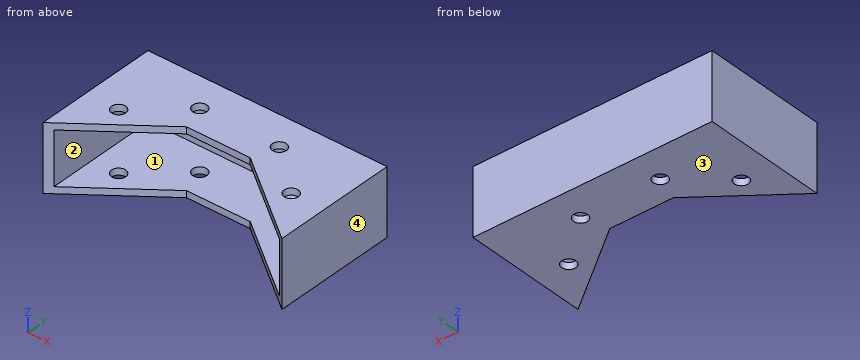
```python
from build123d import *

# Parameters (mm, degrees)
BOSS_EXTRUDE2_DEPTH = 15.875
SHELL2_T            = -3.175
SKETCH3_R           = 3.3782
CUT_EXTRUDE1_DEPTH  = 32.75


with BuildPart() as part:
    # Sketch2 → Boss-Extrude2 (new body, symmetric)
    with BuildSketch(Plane.XY):
        Polygon((-15.24, 0), (15.24, 0), (57.15, -31.75), (57.15, 27.94), (-57.15, 27.94), (-57.15, -31.75), align=None)
    extrude(amount=BOSS_EXTRUDE2_DEPTH, both=True)

    # Shell2
    shell2_openings = [part.faces().sort_by_distance(p)[0] for p in [
        (36.195, -15.875, 0),
        (0, 0, 0),
        (-36.195, -15.875, 0),
    ]]
    offset(amount=SHELL2_T, openings=shell2_openings, kind=Kind.INTERSECTION)

    # Sketch3 → Cut-Extrude1 (cut, through all)
    with BuildSketch(Plane(origin=(0, 0, -15.875), x_dir=(-1, 0, 0), z_dir=(0, 0, -1))):
        with Locations((41.275, -7.62)):
            Circle(SKETCH3_R)
        with Locations((19.05, 12.065)):
            Circle(SKETCH3_R)
        with Locations((-19.05, 12.065)):
            Circle(SKETCH3_R)
        with Locations((-41.275, -7.62)):
            Circle(SKETCH3_R)
    extrude(amount=-CUT_EXTRUDE1_DEPTH, mode=Mode.SUBTRACT)


solid = part.part
```
Can you work these out from the model? Positions are in its coordinate system, mm. Face numbers are marked on the shaded views. Give positions to 0.01 mm unless a question says otherwise; leave off trailing zeros. Order: outer loops, then holes, each group sorted by start corner. A loop starts at its lowest first (then second) coordinate and runs counter-clockwise, first axis right, second up. Notation, with made-up numbers: (42.5, 15.25) - (90.5, 15.25) arc R19 cw to (90.5, 32.25) - close; hole circle Ø9 at (66, 15). An arc over 180 degrees is marked (long way). Use a Markdown table: item, result. Add a question column.
Q1. If we section it at B-B on x = -19.05: Write out the boundary of the cut face in (y, z) (3 decimals), plus the area to 3 significant figures.
Q2. If we section it at D-D on z = -6.5: Write out the boundary of the cut face in (x, y) (3 decimals).
Q3. Please list where these lines run through material, in increasing order: line 1 along X through (y, z) = (-26, -11.5) (3 decimals); line 2 along X through (y, z) = (-7, 15); line 3 along Z through (x, y) = (-39.5, -13) (3 decimals).
Q4. If we mould it in two halves opening along Z, with no side actions, what happens to the marked faces 1, 2, 3 and 4? For each: released by +Z, released by -Z, zero draft, split by the parting line, or undercut.
Q5. If we section it at A-A on y = -25: Write out the boundary of the cut face in (x, z) (3 decimals).
Q6. If we section it at C-C on y = -7.62: Count the separate pieces of the cut face and the enclosed holes in it, plus the area to 3 significant figures.
Q7. I'm going to push flat-ended pins straight in: pin 1 (4 mm diameter, centred on x = 19.05, y = 12.065, fed in from -Z); pin 2 (2.5 mm diameter, centred on x = -2, z = 13.5, fed in from -Y); pin 3 (11 mm diameter, centred on x = 19.05, y = 12.065, fed in from -Z) (3 decimals). Where does each tip first touch, or does it pass through?
Answers follow:
| question | item | result |
|---|---|---|
| 1 | outline | (-2.886, -15.875) - (8.687, -15.875) - (8.687, -12.7) - (-2.886, -12.7) - close; (-2.886, 12.7) - (8.687, 12.7) - (8.687, 15.875) - (-2.886, 15.875) - close; (15.443, -15.875) - (27.94, -15.875) - (27.94, 15.875) - (15.443, 15.875) - (15.443, 12.7) - (24.765, 12.7) - (24.765, -12.7) - (15.443, -12.7) - close |
| 1 | area | 233 mm^2 |
| 2 | outline | (-57.15, -31.75) - (-53.975, -29.345) - (-53.975, 24.765) - (53.975, 24.765) - (53.975, -29.345) - (57.15, -31.75) - (57.15, 27.94) - (-57.15, 27.94) - close |
| 3 | line 1 | x = -57.15 to -53.975, 53.975 to 57.15 |
| 3 | line 2 | x = -57.15 to -44.6, -37.95 to -24.48, 24.48 to 37.95, 44.6 to 57.15 |
| 3 | line 3 | z = -15.875 to -12.7, 12.7 to 15.875 |
| 4 | face 1 | undercut |
| 4 | face 2 | undercut |
| 4 | face 3 | released by -Z |
| 4 | face 4 | zero draft |
| 5 | outline | (-57.15, -15.875) - (-48.24, -15.875) - (-48.24, -12.7) - (-53.975, -12.7) - (-53.975, 12.7) - (-48.24, 12.7) - (-48.24, 15.875) - (-57.15, 15.875) - close; (48.24, -15.875) - (57.15, -15.875) - (57.15, 15.875) - (48.24, 15.875) - (48.24, 12.7) - (53.975, 12.7) - (53.975, -12.7) - (48.24, -12.7) - close |
| 6 | separate pieces | 6 |
| 6 | enclosed holes | 0 |
| 6 | area | 480 mm^2 |
| 7 | pin 1 | passes through |
| 7 | pin 2 | stops at y = 0 |
| 7 | pin 3 | stops at z = -15.875 |
